from build123d import *

# Parameters (mm, degrees)
ESQUISSE2_W                                   = 40
ESQUISSE2_H                                   = 10
BOSS_EXTRU_1_DEPTH                            = 40
DIAM_TRE_DU_PER_AGE_4_1_4_1_1_D               = 4.1
TROU_POUR_TARAUDAGE_POUR_TROU_TARAUD_M6_D     = 5
TROU_POUR_TARAUDAGE_POUR_TROU_TARAUD_M6_DEPTH = 8
TROU_POUR_TARAUDAGE_POUR_TROU_TARAUD_M6_TIP   = 1.502151548
DIAM_TRE_DU_PER_AGE_6_0_6_1_D                 = 6
DIAM_TRE_DU_PER_AGE_6_0_6_1_DEPTH             = 20
DIAM_TRE_DU_PER_AGE_6_0_6_1_TIP               = 1.802581857
TROU_POUR_TARAUDAGE_POUR_TROU_TARAUD_M3_D     = 2.5
TROU_POUR_TARAUDAGE_POUR_TROU_TARAUD_2_D      = 2.5
TROU_POUR_TARAUDAGE_POUR_TROU_TARAUD_2_DEPTH  = 5
TROU_POUR_TARAUDAGE_POUR_TROU_TARAUD_2_TIP    = 0.751075774
CHANFREIN1_SIZE                               = 0.5
ENL_V_START                                   = 8
ESQUISSE20_R                                  = 26.193290648
ESQUISSE20_R_2                                = 5
ENL_V_MAT_EXTRU_1_DEPTH                       = 1.6
R_P_TITION_LIN_AIRE1_COUNT                    = 8
R_P_TITION_LIN_AIRE1_PITCH                    = 3.2


with BuildPart() as part:
    # Esquisse2 → Boss.-Extru.1 (new body)
    with BuildSketch(Plane.XY):
        with Locations((20, 5)):
            Rectangle(ESQUISSE2_W, ESQUISSE2_H)
    extrude(amount=BOSS_EXTRU_1_DEPTH)

    # Diam_tre du per_age _4.1 _4.1_1 (through all)
    with Locations(Plane.XY.offset(40)):
        with Locations((20, 5)):
            Hole(DIAM_TRE_DU_PER_AGE_4_1_4_1_1_D / 2)

    # Trou pour taraudage pour trou taraud_ M6
    with Locations(Plane.XY.offset(40)):
        with Locations((20, 5)):
            Hole(TROU_POUR_TARAUDAGE_POUR_TROU_TARAUD_M6_D / 2, depth=TROU_POUR_TARAUDAGE_POUR_TROU_TARAUD_M6_DEPTH)
            with Locations((0, 0, -(TROU_POUR_TARAUDAGE_POUR_TROU_TARAUD_M6_DEPTH + TROU_POUR_TARAUDAGE_POUR_TROU_TARAUD_M6_TIP / 2))):  # 118° drill point
                Cone(0, TROU_POUR_TARAUDAGE_POUR_TROU_TARAUD_M6_D / 2, TROU_POUR_TARAUDAGE_POUR_TROU_TARAUD_M6_TIP, mode=Mode.SUBTRACT)

    # Diam_tre du per_age _6.0 _6_1
    with Locations(Plane(origin=(0, 0, 0), x_dir=(-1, 0, 0), z_dir=(0, 0, -1))):
        with Locations((-20, 5)):
            Hole(DIAM_TRE_DU_PER_AGE_6_0_6_1_D / 2, depth=DIAM_TRE_DU_PER_AGE_6_0_6_1_DEPTH)
            with Locations((0, 0, -(DIAM_TRE_DU_PER_AGE_6_0_6_1_DEPTH + DIAM_TRE_DU_PER_AGE_6_0_6_1_TIP / 2))):  # 118° drill point
                Cone(0, DIAM_TRE_DU_PER_AGE_6_0_6_1_D / 2, DIAM_TRE_DU_PER_AGE_6_0_6_1_TIP, mode=Mode.SUBTRACT)

    # Trou pour taraudage pour trou taraud_ M3 (through all)
    with Locations(Plane(origin=(0, 0, 0), x_dir=(-1, 0, 0), z_dir=(0, -1, 0))):
        with Locations((-4, -36), (-36, -36), (-36, -4), (-4, -4)):
            Hole(TROU_POUR_TARAUDAGE_POUR_TROU_TARAUD_M3_D / 2)

    # Trou pour taraudage pour trou taraud 2
    with Locations(Plane(origin=(0, 0, 0), x_dir=(-1, 0, 0), z_dir=(0, -1, 0))):
        with Locations((-20, -4)):
            Hole(TROU_POUR_TARAUDAGE_POUR_TROU_TARAUD_2_D / 2, depth=TROU_POUR_TARAUDAGE_POUR_TROU_TARAUD_2_DEPTH)
            with Locations((0, 0, -(TROU_POUR_TARAUDAGE_POUR_TROU_TARAUD_2_DEPTH + TROU_POUR_TARAUDAGE_POUR_TROU_TARAUD_2_TIP / 2))):  # 118° drill point
                Cone(0, TROU_POUR_TARAUDAGE_POUR_TROU_TARAUD_2_D / 2, TROU_POUR_TARAUDAGE_POUR_TROU_TARAUD_2_TIP, mode=Mode.SUBTRACT)

    # Chanfrein1
    chanfrein1_edges = [part.edges().sort_by_distance(p)[0] for p in [
        (40, 5, 40),
        (20, 10, 40),
        (0, 5, 40),
        (20, 10, 0),
        (40, 5, 0),
        (20, 0, 0),
        (0, 5, 0),
        (20, 0, 40),
        (0, 10, 20),
        (40, 10, 20),
        (40, 0, 20),
        (0, 0, 20),
    ]]
    chamfer(chanfrein1_edges, length=CHANFREIN1_SIZE)

    # Esquisse20 → Enl_v. mat.-Extru.1 (cut)
    with BuildSketch(Plane(origin=(0, 40, 40), x_dir=(-1, 0, 0), z_dir=(0, 0, -1)).offset(ENL_V_START)):
        with Locations((-20, -35)):
            Circle(ESQUISSE20_R)
        with Locations(Location((-20, -35, 0), (0, 0, 270))):
            Circle(ESQUISSE20_R_2, mode=Mode.SUBTRACT)
    enl_v_mat_extru_1 = extrude(amount=ENL_V_MAT_EXTRU_1_DEPTH, mode=Mode.SUBTRACT)

    # R_p_tition lin_aire1: Enl_v. mat.-Extru.1 ×8
    with Locations(*[(0, 0, -i * R_P_TITION_LIN_AIRE1_PITCH) for i in range(1, R_P_TITION_LIN_AIRE1_COUNT)]):
        add(enl_v_mat_extru_1, mode=Mode.SUBTRACT)


solid = part.part
The model under review builds one solid part; all positions refer to its coordinate system, in mm. A direction names the side the tool comes from. Give positions to 0.01 mm unless a question says otherwise; leave off trailing zeros. Loops run counter-clockwise (first coordinate to the right, second up) from the corner with the lowest first, then second, coordinate; pieces in that order, holes last. Notation, with made-up numbers: (73.25, 50.5) -> (119.25, 50.5) arc R13 cw to (119.25, 69.5) -> close; hole circle Ø1 at (-12.5, 11). An arc over 180 degrees is marked (long way). Answer as a JSON object with one key per item and string values. Group by question number.
Q1. Tool access review of faces 5 (the flat face through (20, 10, 20)), 6 (the cylindrical face through (24.88, 6.08, 31.21)): name each direction out of +Z, -Z, +X, -X, +Y, -Y from which nothing blocks a thin tool from reaching the whole face with its end or side.
Q2. Insertion check: pin 1 (1.5 mm diameter, centred on x = 22.5, z = 30, fed in from -Y). The pin has a flat end and moves straight along its axis. Give the tip position at first contact, or say it passes through.
Q3. Wall thickness on line 1 along X through (y, z) = (8.25, 36); line 2 along X through (y, z) = (5, 28); line 3 along X through (y, z) = (4, 4): over which ranges is each line inside the solid? List them lowest first.
Q4. Draft analysis for pull direction X (two halves, no side actions). For faces 1 (the cylindrical face through (4.577, 5.07, 37.109)), 2 (the cylindrical face through (22.05, 5.09, 26.07)), 3 (the flat face through (0, 5, 26)), 4 (the flat face through (8, 5, 19.2)), state which applies: pulls with the +X half, pulls with the -X half, needs draft (parallel to the pull), parting line crosses it, or undercut.
Q5. Take a section at C-C (x = 4). State how many separate pieces and enclosed holes the cut face has, plus the area to 4 significant figures.
Q6. Take a section at B-B (z = 6). Write out the cut boundary in (x, y).
Q7. Take a section at A-A (z = 36). Write out the cut boundary in (x, y).
Answer below:
{
 "1": {"face 5": "+Z, -Z, +X, -X, +Y", "face 6": "none"},
 "2": {"pin 1": "stops at y = 0"},
 "3": {"line 1": "x = 0 to 2.75, 5.25 to 34.75, 37.25 to 40", "line 2": "x = 15 to 17.95, 22.05 to 25", "line 3": "x = 0 to 2.75, 5.25 to 17.17, 22.83 to 34.75, 37.25 to 40"},
 "4": {"face 1": "undercut", "face 2": "undercut", "face 3": "pulls with the -X half", "face 4": "needs draft"},
 "5": {"separate pieces": "11", "enclosed holes": "0", "area": "221.5 mm2"},
 "6": {"outline": "(0, 0.5) -> (0.5, 0) -> (39.5, 0) -> (40, 0.5) -> (40, 9.5) -> (39.5, 10) -> (0.5, 10) -> (0, 9.5) -> close; hole circle Ø6 at (20, 5)"},
 "7": {"outline": "(0, 0.5) -> (0.5, 0) -> (2.75, 0) -> (2.75, 10) -> (0.5, 10) -> (0, 9.5) -> close; (5.25, 0) -> (34.75, 0) -> (34.75, 10) -> (5.25, 10) -> close; (37.25, 0) -> (39.5, 0) -> (40, 0.5) -> (40, 9.5) -> (39.5, 10) -> (37.25, 10) -> close; hole circle Ø5 at (20, 5)"}
}
